Autodesk Inventor part; units mm, degrees
ref_plane "Начальная плоскость" through (0, 0, 0) normal (0, 0, 1) x (1, 0, 0)
ref_plane "Конечная плоскость" through (0, 0, 83.315) normal (0, 0, 1) x (1, 0, 0)
ref_plane "РабПлоскость8" through (18, -177.5, 83.315) normal (0, 0, 1) x (1, 0, 0)
ref_plane "Начальная плоскость" through (0, 0, 0) normal (0, 0, 1) x (1, 0, 0)
ref_plane "Конечная плоскость" through (0, 0, 83.315) normal (0, 0, 1) x (1, 0, 0)
sketch "Эскиз" plane through (0, 0, 0) normal (0, 0, 1) x (1, 0, 0)
  line L0 (36, -32.5) -> (0, -32.5)
  line L1 (36, -32.5) -> (36, -28.696)
  line L2 (33.6994, -26.2039) -> (9.9215, -24.3017)
  line L3 (4.4, -18.3208) -> (4.4, 18.3208)
  line L4 (33.6994, 26.2039) -> (9.9215, 24.3017)
  line L5 (36, 28.696) -> (36, 32.5)
  line L6 (0, 32.5) -> (36, 32.5)
  line L7 (0, -32.5) -> (0, 32.5)
  arc A0 (4.4, -18.3208) -> (9.9215, -24.3017) centre (10.4, -18.3208) ccw
  arc A1 (9.9215, 24.3017) -> (4.4, 18.3208) centre (10.4, 18.3208) ccw
  arc A2 (36, -28.696) -> (33.6994, -26.2039) centre (33.5, -28.696) ccw
  arc A3 (33.6994, 26.2039) -> (36, 28.696) centre (33.5, 28.696) ccw
  line L8 (0, 45.5) -> (0, -45.5) construction
  line L9 (-7.2974, 0) -> (43.7847, 0) construction
  point P0 (36, -26.388)
  point P1 (4.4, -23.86)
  point P2 (4.4, 23.86)
  point P3 (36, 26.388)
  dimension "d3" = 36
  dimension "d5" = 4.4
  dimension "d7" = 65
  dimension "d9" = 8.64
  dimension "d11" = 8.64
  dimension "d13" = 6.112
  dimension "d15" = 6.112
  dimension "d22" = 6
  dimension "d23" = 2.5
  dimension "d24" = 32.5
  dimension "d25" = 0
extrude "Тело" add sketch "Эскиз" along normal up to surface (83.315 mm away) from surface at 0
sketch "Sketch3" plane through (0, 0, 0) normal (0, 0, 1) x (1, 0, 0)
  line L0 (0, 0) -> (10, 0)
ref_plane "Work Plane7" through (0, 0, 0) normal (0, -1, 0) x (1, 0, 0)
sketch "Sketch4" plane through (0, 0, 0) normal (0, -1, 0) x (1, 0, 0)
  line L0 (-2, 0) -> (12, 0)
  line L1 (-2, 83.315) -> (12, 83.315)
  dimension "d29" = 83.315
ref_plane "РабПлоскость8" through (18, -177.5, 83.315) normal (0, 0, 1) x (1, 0, 0)
split "Разделение1" plane through (18, -177.5, 83.315) removes the side toward (0, 0, 1)
equation "\"d3\" = b"
equation "\"d7\" = ParH"
equation "\"d22\" = R"
equation "\"d23\" = R1"
equation "\"d24\" = 0.5 * d7"
equation "\"d16\" = G_L"
equation "\"R1\" = 2.5"
equation "\"R\" = 6"
equation "\"t1\" = 4.4"
equation "\"t2\" = 7.2"
equation "\"ParH\" = 65"
equation "\"b\" = 36"
equation "\"msp_x1\" = 0.04 * b"
equation "\"msp_x2\" = -0.08 * t1 + 0.04 * b"
equation "\"G_L\" = d29"
equation "\"ex\" = 0"
equation "\"G_OFFSET_START\" = 0"
equation "\"G_OFFSET_END\" = 0"
equation "\"d27\" = G_OFFSET_END + B_L"
equation "\"B_L\" = 83.315"
properties part number "Швеллер 6.5U-83,32 ГОСТ 8240-97" material "Сталь, мягкая, сварочная"
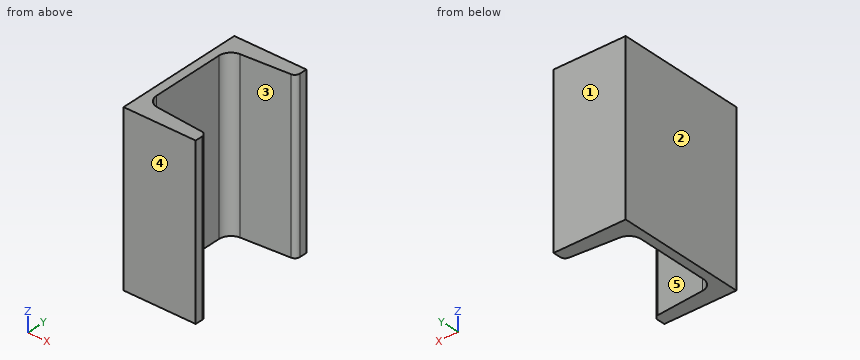
Build history of the part. All positions in model axes, mm. Face numbers are marked on the shaded views. A direction names the side the tool comes from. Coordinates: 2 decimals unless noted, no trailing zeros. Order: outer loops, then holes, each group sorted by start corner. A loop starts at its lowest first (then second) coordinate and runs counter-clockwise, first axis right, second up.
Item 1: Mould opens along Y. For the marked faces 1, 2 and 3 say: released by +Y, released by -Y, zero draft, split by the parting line, or undercut.
Filled in:
face 1: released by +Y
face 2: zero draft
face 3: undercut
Item 2: Saw through at D-D on x = 6. List the corners of the cut face in (y, z) (3 decimals), then the cut area to 3 significant figures.
Filled in:
outline: (-32.5, 0) - (-22.4, 0) - (-22.4, 83.315) - (-32.5, 83.315) - close; (22.4, 0) - (32.5, 0) - (32.5, 83.315) - (22.4, 83.315) - close
area: 1,680 mm2
Item 3: Tool access for the marked faces 4 and 5: list every direction of +Z, -Z, +X, -X, +Y, -Y with a clear straight run to the whole face (end or side of a thin tool).
Filled in:
face 4: +Z, -Z, +X, -X, -Y
face 5: +Z, -Z, +X
Item 4: Drop flat-ended pins along their axis: pin 1 Ø4 at (y, z) = (-21.5, 48) entering from +X; pin 2 Ø12 at (y, z) = (-12.5, 41.5) entering from +X. Give the stop position or say it passes through.
Filled in:
pin 1: stops at x = 7.37
pin 2: stops at x = 4.4
Item 5: Saw through at B-B on z = 11. List the corners of the cut face in (x, y), then the cut area to 3 significant figures.
Filled in:
outline: (0, -32.5) - (36, -32.5) - (36, -28.7) arc R2.5 ccw to (33.7, -26.2) - (9.92, -24.3) arc R6 cw to (4.4, -18.32) - (4.4, 18.32) arc R6 cw to (9.92, 24.3) - (33.7, 26.2) arc R2.5 ccw to (36, 28.7) - (36, 32.5) - (0, 32.5) - close
area: 763 mm2
Item 6: Saw through at A-A on x = 31. List the corners of the cut face in (y, z) (3 decimals), then the cut area to 3 significant figures.
Filled in:
outline: (-32.5, 0) - (-25.988, 0) - (-25.988, 83.315) - (-32.5, 83.315) - close; (25.988, 0) - (32.5, 0) - (32.5, 83.315) - (25.988, 83.315) - close
area: 1,090 mm2
Item 7: Drill centre lines: L1, parallel to X at y = 2, z = 13; L2, parallel to Y at x = 14, z = 21; L3, parallel to Y at x = 32.5, z = 21. Where is each one in solid material? Low to high.
Filled in:
L1: x = 0 to 4.4
L2: y = -32.5 to -24.63, 24.63 to 32.5
L3: y = -32.5 to -26.11, 26.11 to 32.5
Item 8: Saw through at C-C on y = -1.5. List the corners of the cut face in (x, z) (3 decimals), then the cut area to 3 significant figures.
Filled in:
outline: (0, 0) - (4.4, 0) - (4.4, 83.315) - (0, 83.315) - close
area: 367 mm2
